Print and shaded views of the part. All mm, measured from the part's lowest x, y and z. A direction names the side the tool comes from. Coordinates: 2 decimals unless noted, no trailing zeros. Order: outer loops, then holes, each group sorted by start corner. A loop starts at its lowest first (then second) coordinate and runs counter-clockwise, first axis right, second up.
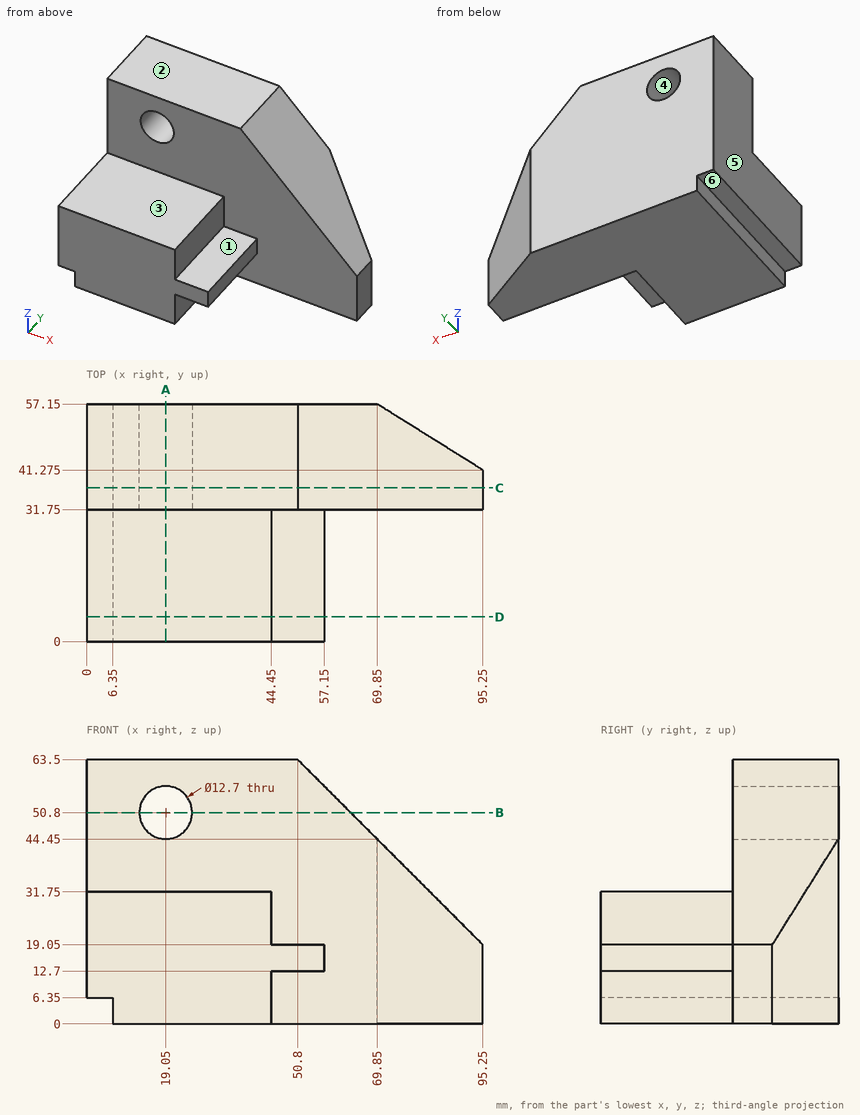
Q1. Cut at A-A, the plane x = 19.05. List the corners of the cut face in (y, z), plus the area to 3 significant figures.
Established:
outline: (0, 0) - (57.15, 0) - (57.15, 44.45) - (31.75, 44.45) - (31.75, 31.75) - (0, 31.75) - close; (31.75, 57.15) - (57.15, 57.15) - (57.15, 63.5) - (31.75, 63.5) - close
area: 2,300 mm2
Q2. Which spindle directions (+Z, -Z, +X, -X, +Y, -Y) get a long thin tool onto all of the face, cutting with end or side? Do the marked faces 1, 2 and 3. Say none if no direction does.
Established:
face 1: +Z, +X, -Y
face 2: +Z, +X, -X, +Y, -Y
face 3: +Z, +X, -X, -Y
Q3. Cut at B-B, the plane z = 50.8. List the corners of the cut face in (x, y), plus the area to 3 significant figures.
Established:
outline: (0, 31.75) - (12.7, 31.75) - (12.7, 57.15) - (0, 57.15) - close; (25.4, 31.75) - (63.5, 31.75) - (63.5, 57.15) - (25.4, 57.15) - close
area: 1,290 mm2
Q4. Mould opens along X. For the marked faces 4, 5 and 6 say: pulls with the +X half, pulls with the -X half, needs draft (parallel to the pull), parting line crosses it, or undercut.
Established:
face 4: undercut
face 5: pulls with the -X half
face 6: needs draft
Q5. Cut at D-D, the plane y = 6. List the corners of the cut face in (x, z).
Established:
outline: (0, 6.35) - (6.35, 6.35) - (6.35, 0) - (44.45, 0) - (44.45, 12.7) - (57.15, 12.7) - (57.15, 19.05) - (44.45, 19.05) - (44.45, 31.75) - (0, 31.75) - close
Q6. Probe line 1 (Z direction, x = 19.05, y = 51); line 2 (Y direction, x = 52.5, z = 20.5); line 3 (X direction, y = 17.5, z = 30). List the from-to ranges inside material, lowest first.
Established:
line 1: z = 0 to 44.45, 57.15 to 63.5
line 2: y = 31.75 to 57.15
line 3: x = 0 to 44.45
Q7. Drop flat-ended pins along their axis: P1, Ø3, axis at y = 17.5, z = 15.5, coming from the +X side; P2, Ø1, axis at x = 79.5, z = 20, coming from the +Y side; P3, Ø6.5, axis at x = 51, y = 8.5, coming from the +Z side; P4, Ø1, axis at x = 71.5, z = 45.5, coming from the -Y side. Give the stop position or say it passes through.
Established:
P1: stops at x = 57.15
P2: stops at y = 51.43
P3: stops at z = 19.05
P4: passes through
Q8. Cut at C-C, the plane y = 37. List the corners of the cut face in (x, z).
Established:
outline: (0, 6.35) - (6.35, 6.35) - (6.35, 0) - (95.25, 0) - (95.25, 19.05) - (50.8, 63.5) - (0, 63.5) - close; hole circle Ø12.7 at (19.05, 50.8)
